Could you check a few things on this model? Use its own coordinates, in mm. Give positions to 0.01 mm unless a question says otherwise; leave off trailing zeros. Loops run counter-clockwise (first coordinate to the right, second up) from the corner with the lowest first, then second, coordinate; pieces in that order, holes last. Notation, with made-up numbers: (7, 74) - (39, 74) arc R18 ccw to (39, 105) - close; hole circle Ø3 at (89.5, 54.5). An arc over 180 degrees is marked (long way). Write each question's results on one line, items separated by ' | '. Start each with the question number.
1) I'm going to push flat-ended pins straight in: pin 1 (1.9 mm diameter, centred on x = 33.1, y = 16.9, fed in from +Z); pin 2 (2 mm diameter, centred on x = 35, z = 56.5, fed in from +Y); pin 3 (4 mm diameter, centred on x = 35.5, y = 46.5, fed in from -Z); pin 4 (4 mm diameter, centred on x = 32.5, y = 15.5, fed in from -Z). Where does each tip first touch, or does it pass through?
2) I want a section at A-A, the plane y = 37. Write out the boundary of the cut face in (x, z), and give its area (4 significant figures).
3) I want a section at B-B, the plane z = 39.5. Write out the boundary of the cut face in (x, y), and give its area (3 significant figures).
4) If I drill on probe 1 along Y at (x, z) = (37.5, 39); probe 2 along X at (y, z) = (19, 51); probe 3 along Z at (x, y) = (37, 28), over which ranges is the centre line in solid material (lowest first)? Write a range as [from, to].
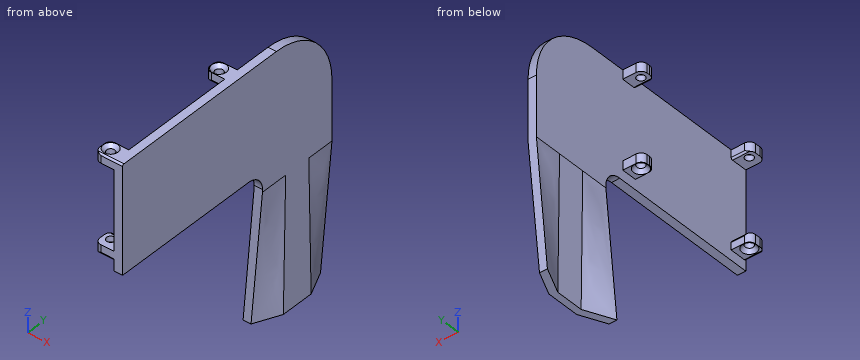
from build123d import *
from OCP.BRepFilletAPI import BRepFilletAPI_MakeFillet

# Parameters (mm, degrees)
BOSS_EXTRUDE1_START                                 = 0.25
SKETCH1_W                                           = 2.7
SKETCH1_H                                           = 4.5
BOSS_EXTRUDE1_DEPTH                                 = 5.8
SKETCH1_H_2                                         = 5.25
BOSS_EXTRUDE1_2_DEPTH                               = 5.8
BOSS_EXTRUDE1_3_DEPTH                               = 5.8
BOSS_EXTRUDE1_4_DEPTH                               = 5.8
SKETCH2_W                                           = 32.1
SKETCH2_H                                           = 44.25
BOSS_EXTRUDE2_DEPTH                                 = 2.5
BOSS_EXTRUDE3_DEPTH                                 = 2.5
CSK_FOR_M2_COUNTERSUNK_FLAT_HEAD_SCREW1_D           = 2.4
CSK_FOR_M2_COUNTERSUNK_FLAT_HEAD_SCREW1_DEPTH       = 4
CSK_FOR_M2_COUNTERSUNK_FLAT_HEAD_SCREW1_CSINK_D     = 4.4
CSK_FOR_M2_COUNTERSUNK_FLAT_HEAD_SCREW1_CSINK_ANGLE = 90
CSK_FOR_M2_COUNTERSUNK_FLAT_HEAD_SCREW1_TIP         = 0.721032743
CSK_FOR_M2_COUNTERSUNK_FLAT_HEAD_SCREW2_D           = 2.4
CSK_FOR_M2_COUNTERSUNK_FLAT_HEAD_SCREW2_DEPTH       = 4
CSK_FOR_M2_COUNTERSUNK_FLAT_HEAD_SCREW2_CSINK_D     = 4.4
CSK_FOR_M2_COUNTERSUNK_FLAT_HEAD_SCREW2_CSINK_ANGLE = 90
CSK_FOR_M2_COUNTERSUNK_FLAT_HEAD_SCREW2_TIP         = 0.721032743
FILLET1_R1                                          = 20
FILLET1_R2                                          = 5
FILLET2_R                                           = 1.8
FILLET3_R                                           = 0.5


with BuildPart() as part:
    # Sketch1 → Boss-Extrude1 (new body)
    with BuildSketch(Plane(origin=(30.600472417, 0, 0), x_dir=(0, 0, -1), z_dir=(1, 0, 0)).offset(BOSS_EXTRUDE1_START)):
        with Locations((-30.576835801, 55.903969126)):
            Rectangle(SKETCH1_W, SKETCH1_H)
    extrude(amount=BOSS_EXTRUDE1_DEPTH)



with BuildPart() as body_2:
    # Sketch1 → Boss-Extrude1 2 (new body)
    with BuildSketch(Plane(origin=(30.600472417, 0, 0), x_dir=(0, 0, -1), z_dir=(1, 0, 0)).offset(BOSS_EXTRUDE1_START)):
        with Locations((-30.576835801, 16.528969126)):
            Rectangle(SKETCH1_W, SKETCH1_H_2)
    extrude(amount=BOSS_EXTRUDE1_2_DEPTH)


with BuildPart() as body_3:
    # Sketch1 → Boss-Extrude1 3 (new body)
    with BuildSketch(Plane(origin=(30.600472417, 0, 0), x_dir=(0, 0, -1), z_dir=(1, 0, 0)).offset(BOSS_EXTRUDE1_START)):
        with Locations((-56.976835801, 16.528969126)):
            Rectangle(SKETCH1_W, SKETCH1_H_2)
    extrude(amount=BOSS_EXTRUDE1_3_DEPTH)


with BuildPart() as body_4:
    # Sketch1 → Boss-Extrude1 4 (new body)
    with BuildSketch(Plane(origin=(30.600472417, 0, 0), x_dir=(0, 0, -1), z_dir=(1, 0, 0)).offset(BOSS_EXTRUDE1_START)):
        with Locations((-56.976835801, 55.903969126)):
            Rectangle(SKETCH1_W, SKETCH1_H)
    extrude(amount=BOSS_EXTRUDE1_4_DEPTH)


with BuildPart() as part_1:
    add(part.part)

    add(body_2.part)  # Boss-Extrude2 merges body 2

    add(body_3.part)  # Boss-Extrude2 merges body 3

    add(body_4.part)  # Boss-Extrude2 merges body 4
    # Sketch2 → Boss-Extrude2 (add)
    with BuildSketch(Plane(origin=(36.650472417, 0, 0), x_dir=(0, 0, -1), z_dir=(1, 0, 0))):
        with Locations((-42.276835801, 36.028969126)):
            Rectangle(SKETCH2_W, SKETCH2_H)
    extrude(amount=BOSS_EXTRUDE2_DEPTH)

    # Sketch3 → Boss-Extrude3 (add)
    with BuildSketch(Plane(origin=(39.150472417, 0, 0), x_dir=(0, 0, -1), z_dir=(1, 0, 0))):
        Polygon((-20.426835801, 89.232146542), (-58.326835801, 89.232146542), (-58.326835801, 58.153969126), (-26.226835801, 58.153969126), (-26.226835801, 64.232146542), (-20.426835801, 64.232146542), align=None)
    extrude(amount=-BOSS_EXTRUDE3_DEPTH)

    # CSK for M2 Countersunk Flat Head Screw1
    with Locations(Plane.XY.offset(58.326835801)):
        with Locations((33.100472417, 55.903969126), (33.100472417, 16.903969126)):
            CounterSinkHole(CSK_FOR_M2_COUNTERSUNK_FLAT_HEAD_SCREW1_D / 2, CSK_FOR_M2_COUNTERSUNK_FLAT_HEAD_SCREW1_CSINK_D / 2, depth=CSK_FOR_M2_COUNTERSUNK_FLAT_HEAD_SCREW1_DEPTH, counter_sink_angle=CSK_FOR_M2_COUNTERSUNK_FLAT_HEAD_SCREW1_CSINK_ANGLE)
            with Locations((0, 0, -(CSK_FOR_M2_COUNTERSUNK_FLAT_HEAD_SCREW1_DEPTH + CSK_FOR_M2_COUNTERSUNK_FLAT_HEAD_SCREW1_TIP / 2))):  # 118° drill point
                Cone(0, CSK_FOR_M2_COUNTERSUNK_FLAT_HEAD_SCREW1_D / 2, CSK_FOR_M2_COUNTERSUNK_FLAT_HEAD_SCREW1_TIP, mode=Mode.SUBTRACT)

    # CSK for M2 Countersunk Flat Head Screw2
    with Locations(Plane(origin=(0, 0, 29.226835801), x_dir=(-1, 0, 0), z_dir=(0, 0, -1))):
        with Locations((-33.100472417, 55.903969126), (-33.100472417, 16.903969126)):
            CounterSinkHole(CSK_FOR_M2_COUNTERSUNK_FLAT_HEAD_SCREW2_D / 2, CSK_FOR_M2_COUNTERSUNK_FLAT_HEAD_SCREW2_CSINK_D / 2, depth=CSK_FOR_M2_COUNTERSUNK_FLAT_HEAD_SCREW2_DEPTH, counter_sink_angle=CSK_FOR_M2_COUNTERSUNK_FLAT_HEAD_SCREW2_CSINK_ANGLE)
            with Locations((0, 0, -(CSK_FOR_M2_COUNTERSUNK_FLAT_HEAD_SCREW2_DEPTH + CSK_FOR_M2_COUNTERSUNK_FLAT_HEAD_SCREW2_TIP / 2))):  # 118° drill point
                Cone(0, CSK_FOR_M2_COUNTERSUNK_FLAT_HEAD_SCREW2_D / 2, CSK_FOR_M2_COUNTERSUNK_FLAT_HEAD_SCREW2_TIP, mode=Mode.SUBTRACT)

    # Fillet1: one fillet with a radius per group of edges: ONE call of the kernel's fillet builder (fillet() takes one radius for all edges)
    fillet1_edges_1 = [part_1.edges().sort_by_distance(p)[0] for p in [
        (37.900472417, 89.232146542, 58.326835801),
    ]]
    fillet1_edges_2 = [part_1.edges().sort_by_distance(p)[0] for p in [
        (37.900472417, 64.232146542, 26.226835801),
    ]]
    fillet1 = BRepFilletAPI_MakeFillet(part_1.part.solid().wrapped)
    for e in fillet1_edges_1:
        fillet1.Add(FILLET1_R1, e.wrapped)
    for e in fillet1_edges_2:
        fillet1.Add(FILLET1_R2, e.wrapped)
    add(Compound.cast(fillet1.Shape()), mode=Mode.REPLACE)

    # Loft1: read off the stored shape, not the designer's step
    # Loft1: loft between two sections, ruled curve by curve
    loft1_from = [
        Edge.make_bspline([(39.150472417, 81.726792839, -19.573164199), (38.579023668, 82.977685123, -19.573164199), (38.007574919, 84.228577407, -19.573164199), (36.864677421, 86.730361975, -19.573164199), (36.293228672, 87.981254258, -19.573164199), (35.721779923, 89.232146542, -19.573164199)], [0, 0, 0, 0, 0.5, 0.5, 1, 1, 1, 1], 3),
        Edge.make_bspline([(33.358759351, 89.232146542, -19.573164199), (33.990711529, 87.848813209, -19.573164199), (34.622663707, 86.465479876, -19.573164199), (35.886568062, 83.698813209, -19.573164199), (36.51852024, 82.315479876, -19.573164199), (37.150472417, 80.932146542, -19.573164199)], [0, 0, 0, 0, 0.5, 0.5, 1, 1, 1, 1], 3),
        Edge.make_bspline([(37.150472417, 72.532146542, -19.573164199), (36.51852024, 71.148813209, -19.573164199), (35.886568062, 69.765479876, -19.573164199), (34.622663707, 66.998813209, -19.573164199), (33.990711529, 65.615479876, -19.573164199), (33.358759351, 64.232146542, -19.573164199)], [0, 0, 0, 0, 0.5, 0.5, 1, 1, 1, 1], 3),
        Edge.make_bspline([(35.721779923, 64.232146542, -19.573164199), (36.293228672, 65.483038826, -19.573164199), (36.864677421, 66.73393111, -19.573164199), (38.007574919, 69.235715678, -19.573164199), (38.579023668, 70.486607962, -19.573164199), (39.150472417, 71.737500246, -19.573164199)], [0, 0, 0, 0, 0.5, 0.5, 1, 1, 1, 1], 3),
        Edge.make_line((37.150472417, 72.532146542, -19.573164199), (37.150472417, 80.932146542, -19.573164199)),
        Edge.make_line((33.358759351, 89.232146542, -19.573164199), (35.721779923, 89.232146542, -19.573164199)),
        Edge.make_line((35.721779923, 64.232146542, -19.573164199), (33.358759351, 64.232146542, -19.573164199)),
        Edge.make_line((39.150472417, 71.737500246, -19.573164199), (39.150472417, 81.726792839, -19.573164199)),
    ]
    loft1_to = [
        Edge.make_bspline([(39.150472417, 80.898813209, 20.426835801), (39.150472417, 82.287702098, 20.426835801), (39.150472417, 83.676590987, 20.426835801), (39.150472417, 86.454368765, 20.426835801), (39.150472417, 87.843257653, 20.426835801), (39.150472417, 89.232146542, 20.426835801)], [0, 0, 0, 0, 0.5, 0.5, 1, 1, 1, 1], 3),
        Edge.make_bspline([(36.650472417, 89.232146542, 20.426835801), (36.650472417, 87.843257653, 20.426835801), (36.650472417, 86.454368765, 20.426835801), (36.650472417, 83.676590987, 20.426835801), (36.650472417, 82.287702098, 20.426835801), (36.650472417, 80.898813209, 20.426835801)], [0, 0, 0, 0, 0.5, 0.5, 1, 1, 1, 1], 3),
        Edge.make_bspline([(36.650472417, 72.565479876, 20.426835801), (36.650472417, 71.176590987, 20.426835801), (36.650472417, 69.787702098, 20.426835801), (36.650472417, 67.00992432, 20.426835801), (36.650472417, 65.621035431, 20.426835801), (36.650472417, 64.232146542, 20.426835801)], [0, 0, 0, 0, 0.5, 0.5, 1, 1, 1, 1], 3),
        Edge.make_bspline([(39.150472417, 64.232146542, 20.426835801), (39.150472417, 65.621035431, 20.426835801), (39.150472417, 67.00992432, 20.426835801), (39.150472417, 69.787702098, 20.426835801), (39.150472417, 71.176590987, 20.426835801), (39.150472417, 72.565479876, 20.426835801)], [0, 0, 0, 0, 0.5, 0.5, 1, 1, 1, 1], 3),
        Edge.make_line((36.650472417, 72.565479876, 20.426835801), (36.650472417, 80.898813209, 20.426835801)),
        Edge.make_line((36.650472417, 89.232146542, 20.426835801), (39.150472417, 89.232146542, 20.426835801)),
        Edge.make_line((39.150472417, 64.232146542, 20.426835801), (36.650472417, 64.232146542, 20.426835801)),
        Edge.make_line((39.150472417, 72.565479876, 20.426835801), (39.150472417, 80.898813209, 20.426835801)),
    ]
    loft1 = Solid(Shell([*[Face.make_surface_from_curves(loft1_from[k], loft1_to[k]) for k in range(8)], Face(Wire(loft1_from)), Face(Wire(loft1_to))]))
    add(loft1)

    # Fillet2
    fillet2_edges = [part_1.edges().sort_by_distance(p)[0] for p in [
        (30.850472417, 58.153969126, 30.576835801),
        (30.850472417, 13.903969126, 30.576835801),
        (30.850472417, 53.653969126, 30.576835801),
        (30.850472417, 19.153969126, 30.576835801),
        (30.850472417, 19.153969126, 56.976835801),
        (30.850472417, 13.903969126, 56.976835801),
        (30.850472417, 58.153969126, 56.976835801),
        (30.850472417, 53.653969126, 56.976835801),
    ]]
    fillet(fillet2_edges, radius=FILLET2_R)

    # Fillet3
    # the kernel refuses this fillet: 0.5 mm, written as the material it takes off along each edge
    with BuildSketch(Plane(origin=(40.400472417, 13.903969126, 58.326835801), x_dir=(0, 1, 0), z_dir=(-1, 0, 0))) as fillet3_piece_1:
        with BuildLine():
            CenterArc((FILLET3_R, FILLET3_R), FILLET3_R, 180, 90)
            Line((0, FILLET3_R), (0, 0))
            Line((0, 0), (FILLET3_R, 0))
        make_face()
    extrude(amount=9, mode=Mode.SUBTRACT)
    with BuildSketch(Plane(origin=(31.400472417, 19.153969126, 31.926835801), x_dir=(0, -1, 0), z_dir=(1, 0, 0)), Plane(origin=(31.400472417, 19.153969126, 55.626835801), x_dir=(0, 0, 1), z_dir=(1, 0, 0)), Plane(origin=(31.400472417, 53.653969126, 31.926835801), x_dir=(0, 0, -1), z_dir=(1, 0, 0))) as fillet3_piece_2:
        with BuildLine():
            CenterArc((FILLET3_R, FILLET3_R), FILLET3_R, 180, 90)
            Line((0, FILLET3_R), (0, 0))
            Line((0, 0), (FILLET3_R, 0))
        make_face()
    extrude(amount=5.25, mode=Mode.SUBTRACT)
    with BuildSketch(Plane(origin=(31.400472417, 13.903969126, 29.226835801), x_dir=(0, 0, 1), z_dir=(1, 0, 0)), Plane(origin=(31.400472417, 53.653969126, 55.626835801), x_dir=(0, 0, 1), z_dir=(1, 0, 0))) as fillet3_piece_3:
        with BuildLine():
            CenterArc((FILLET3_R, -FILLET3_R), FILLET3_R, 90, 90)
            Line((0, -FILLET3_R), (0, 0))
            Line((0, 0), (FILLET3_R, 0))
        make_face()
    extrude(amount=5.25, mode=Mode.SUBTRACT)


solid = part_1.part
Answers:
1) pin 1: passes through | pin 2: stops at y = 58.15 | pin 3: stops at z = 26.23 | pin 4: stops at z = 29.23
2) outline: (36.65, 26.23) - (39.15, 26.23) - (39.15, 58.33) - (36.65, 58.33) - close | area: 80.25 mm2
3) outline: (36.65, 13.9) - (39.15, 13.9) - (39.15, 89.2) - (36.65, 89.2) - close | area: 188 mm2
4) probe 1: y = [13.9, 89.22] | probe 2: x = [36.65, 39.15] | probe 3: z = [26.23, 58.33]
